Verification items for this drawing (mm, ordinates from the low corner). A direction names the side the tool comes from. Round coordinates to 2 decimals unless told otherwise and drop trailing zeros. Order: outer loops, then holes, each group sorted by start corner. A loop starts at its lowest first (then second) coordinate and runs counter-clockwise, first axis right, second up. Notation, with made-up numbers: (31, 43) -> (59, 43) arc R21 cw to (59, 69) -> close; hole circle Ø4 at (78, 12). An arc over 180 degrees is marked (long way). Use a Markdown table: item, result. Add a question column.
Item 1: Sectioned sample at A-A, the plane z = 116.84. Record the cut outline in (x, y), and give its area (3 significant figures).
Item 2: Mould release check, pull along Y, two halves, no side actions. Record for the marked faces 1, 2 and 3: pulls with the +Y half, pulls with the -Y half, needs draft (parallel to the pull), parting line crosses it, or undercut.
Item 3: Material ranges on probe 1 along Z at (x, y) = (116, 49); probe 2 along Y at (x, z) = (140.5, 116.84), recorded low to high. Write a range as [from, to].
Item 4: Sectioned sample at B-B, the plane x = 100.5. Record the cut outline in (y, z) (1 decimal), and give its area (3 significant figures).
Item 5: Gauge pin test, flat ends, axial feed: pin 1 Ø5 at (x, z) = (172.5, 203) entering from +Y; pin 2 Ø6 at (y, z) = (123.5, 24) entering from -X; pin 3 Ø3 at (x, y) = (33, 108.5) entering from -Z. Record the tip position at first contact, or that the pin passes through.
Item 6: Sectioned sample at C-C, the plane y = 260. Record the cut outline in (x, z) (3 decimals).
Item 7: Set-up check for the marked faces 4 and 5: record each of +Z, -Z, +X, -X, +Y, -Y from which the full face is reachable in a straight line by a thin tool's end or side.
Item 8: Sectioned sample at D-D, the plane x = 181.5. Record the cut outline in (y, z) (1 decimal).
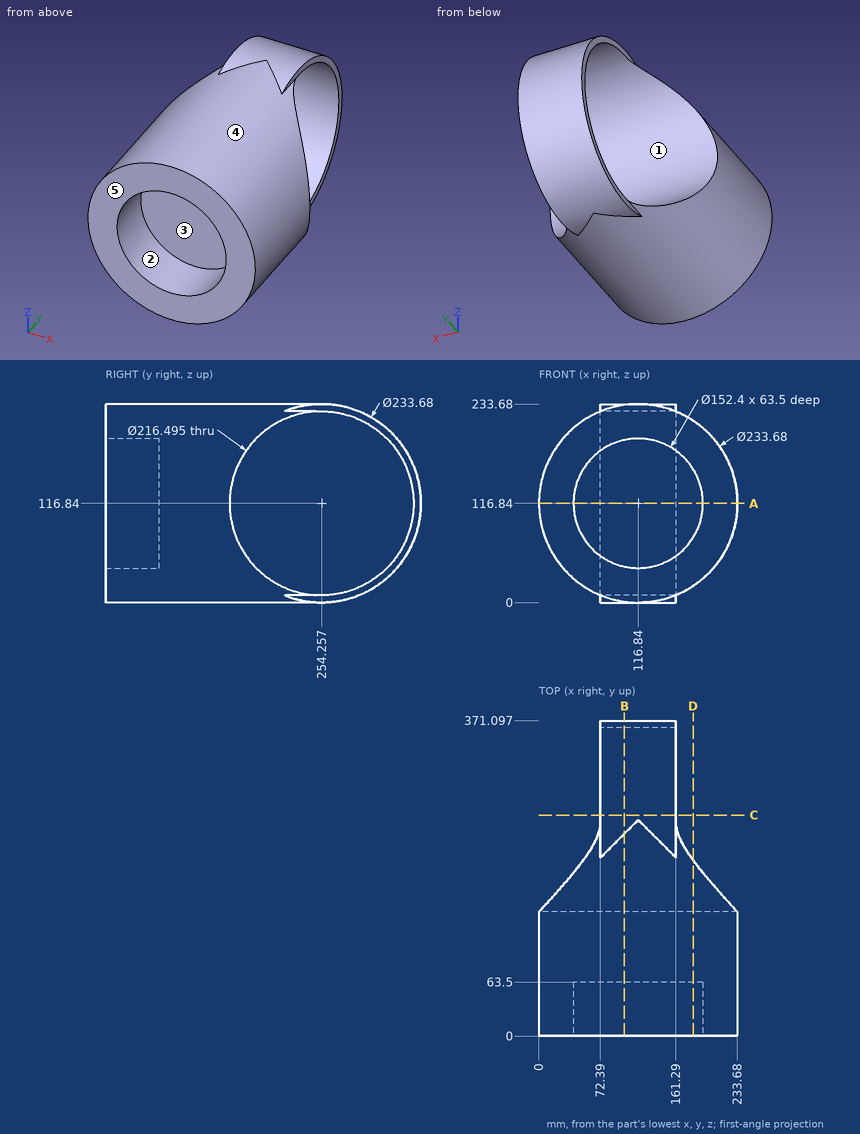
Found:
| question | item | result |
|---|---|---|
| 1 | outline | (0, 0) -> (40.64, 0) -> (40.64, 63.5) -> (193.04, 63.5) -> (193.04, 0) -> (233.68, 0) -> (233.68, 146.01) -> (0, 146.01) -> close; (72.39, 362.5) -> (161.29, 362.5) -> (161.29, 371.1) -> (72.39, 371.1) -> close |
| 1 | area | 25,200 mm2 |
| 2 | face 1 | undercut |
| 2 | face 2 | needs draft |
| 2 | face 3 | pulls with the -Y half |
| 3 | probe 1 | z = [0, 40.64], [193.04, 233.68] |
| 3 | probe 2 | y = [63.5, 146.01], [362.5, 371.1] |
| 4 | outline | (0, 1.1) -> (237.9, 1.1) arc R116.8 ccw (long way) to (237.9, 232.5) -> (0, 232.5) -> (0, 191.3) -> (63.5, 191.3) -> (63.5, 42.4) -> (0, 42.4) -> close; hole circle Ø216.5 at (254.3, 116.8) |
| 4 | area | 34,000 mm2 |
| 5 | pin 1 | stops at y = 192.15 |
| 5 | pin 2 | stops at x = 42.14 |
| 5 | pin 3 | stops at z = 33.94 |
| 6 | outline | (72.39, 0.141) -> (161.29, 0.141) -> (161.29, 8.745) -> (72.39, 8.745) -> close; (72.39, 224.935) -> (161.29, 224.935) -> (161.29, 233.539) -> (72.39, 233.539) -> close |
| 7 | face 4 | -Y |
| 7 | face 5 | +Z, -Z, +X, -X, -Y |
| 8 | outline | (0, 19.5) -> (206.9, 19.5) arc R108.2 cw to (206.9, 214.2) -> (0, 214.2) -> (0, 157.2) -> (63.5, 157.2) -> (63.5, 76.5) -> (0, 76.5) -> close |
